Autodesk Inventor part; units mm, degrees
ref_plane "YZ Plane" through (0, 0, 0) normal (1, 0, 0) x (0, 1, 0)
ref_plane "XZ Plane" through (0, 0, 0) normal (0, 1, 0) x (-1, 0, 0)
ref_plane "XY Plane" through (0, 0, 0) normal (0, 0, 1) x (1, 0, 0)
sketch "Эскиз1" plane through (0, 0, 0) normal (0, 1, 0) x (-1, 0, 0)
  line L0 (0, 0) -> (3, 0)
  line L1 (3, 0) -> (3, -3)
  line L2 (0, -3) -> (1.5, -3)
  line L3 (1.5, -6) -> (1.5, -19)
  line L4 (1.5, -19) -> (0, -19)
  line L5 (0, -19) -> (0, 0)
  line L6 (1.5, -3) -> (3, -3)
  line L7 (1.5, -3) -> (2, -3)
  line L8 (2, -3) -> (2, -6)
  line L9 (2, -6) -> (0, -6)
  dimension "d0" = 3
  dimension "d1" = 3
  dimension "d2" = 1.5
  dimension "d3" = 16
  dimension "d4" = 0.5
  dimension "d5" = 3
revolve "Вращение1" add sketch "Эскиз1" angle 360 about axis through (0, 0, -19) along (0, 0, 1)
thread "Резьба1"
chamfer "Фаска1" distance 0.5 angle 45 1 edges at (1.5, 0, -19)
properties part number "Болт М3х16"
The model under review builds one solid part; all positions refer to its coordinate system, in mm. A direction names the side the tool comes from. Coordinates: 2 decimals unless noted, no trailing zeros. Write each loop counter-clockwise with the first axis right and the second up, starting at its lowest first coordinate (ties: lowest second). Pieces come first, ordered by that corner, then holes. Notation, with made-up numbers: (10, 31) -> (17, 31) arc R26 cw to (17, 60) -> close; hole circle Ø4 at (37, 80.25). An arc over 180 degrees is marked (long way). One line per item, written item: value. Start each with the question number.
Q1. Add section C-C, the plane z = -3.75. Give the boundary of the cut face in (x, y).
Q2. Clearance check with a flat-ended pin moving along its axis: P1, Ø2, axis at x = 0, z = -4.5, coming from the -Y side. State where the tip first meets the part, or that it passes through.
Q3. Add section D-D, the plane y = -1.7. Give the boundary of the cut face in (x, z), then the cut area to 3 significant figures.
Q4. To check wall thickness, follow probe 1 along Z at (x, y) = (-1.3, 1.6); probe 2 along Z at (x, y) = (-0.6, -1.85); probe 3 along Y at (x, z) = (-0.1, -2.75). State the ranges of each line that lie inside material, in increasing order.
Q5. Add section A-A, the plane x = 0. Give the boundary of the cut face in (y, z), then the cut area to 4 significant figures.
Q6. For faces 1 (the face through (3, 0, -2)), 2 (the face through (1.5, 0.07, -12.34)), list the 3-axis set-ups (+Z, -Z, +X, -X, +Y, -Y) from which the entire face can be reached by the end or side of a thin tool; tool diameter is ignored.
Response:
1. outline: circle Ø4 at (0, 0)
2. P1: y = -2
3. outline: (-2.47, -3) -> (-1.05, -3) -> (-1.05, -6) -> (1.05, -6) -> (1.05, -3) -> (2.47, -3) -> (2.47, 0) -> (-2.47, 0) -> close
3. area: 21.2 mm²
4. probe 1: -3 to 0
4. probe 2: -6 to 0
4. probe 3: -3 to 3
5. outline: (-3, -3) -> (-2, -3) -> (-2, -6) -> (-1.5, -6) -> (-1.5, -18.5) -> (-1, -19) -> (1, -19) -> (1.5, -18.5) -> (1.5, -6) -> (2, -6) -> (2, -3) -> (3, -3) -> (3, 0) -> (-3, 0) -> close
5. area: 68.75 mm²
6. face 1: +Z, -Z
6. face 2: -Z
